For this review, use the dimensioned drawing (mm, ordinates from the lowest corner) and the shaded views. Give positions to 0.01 mm unless a question says otherwise; leave off trailing zeros. Loops run counter-clockwise (first coordinate to the right, second up) from the corner with the lowest first, then second, coordinate; pieces in that order, holes last. Notation, with made-up numbers: (35, -22.75) -> (58, -22.75) arc R16 cw to (58, -7.75) -> close; hole circle Ø11 at (41, -37). An arc over 180 degrees is marked (long way). Use a Markdown table: item, result. Add a question column.
1. For pin 1 Ø2 at (y, z) = (3, 0.5) entering from -X; pin 2 Ø1.5 at (x, z) = (3, 3) entering from -Y; pin 3 Ø2 at (y, z) = (4, 2.5) entering from -X, all flat-tipped, find the tip position at first contact; note any pin that passes through.
2. Add section C-C (z = 2.25). State the section outline as (x, y) points, and give its area (3 significant figures).
3. Add section A-A (y = 6.75). State the section outline as (x, z) points, and give its area (3 significant figures).
4. Draft analysis for pull direction Y (two halves, no side actions). For the marked faces 1, 2 and 3, state which applies: pulls with the +Y half, pulls with the -Y half, needs draft (parallel to the pull), parting line crosses it, or undercut.
5. To check wall thickness, follow line 1 (Y direction, x = 6.75, z = 1.55); line 2 (Y direction, x = 9.5, z = 3.25); line 3 (X direction, y = 5.75, z = 3.05). State the ranges of each line that lie inside material, in increasing order.
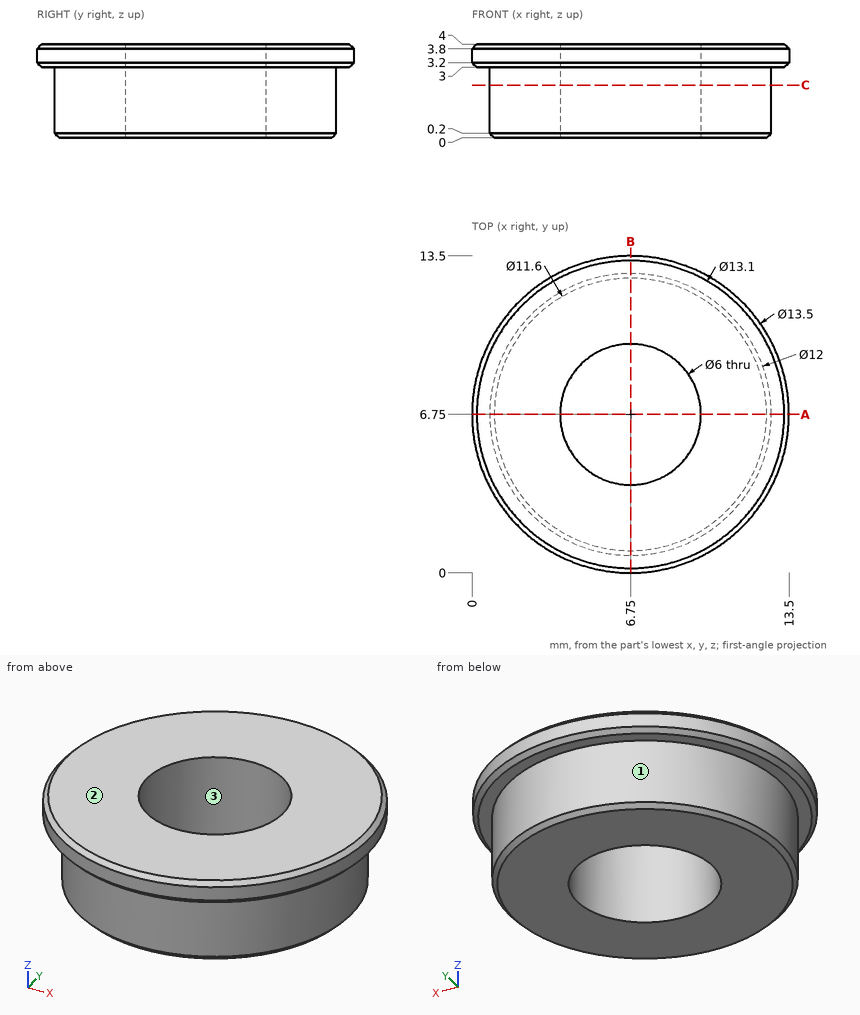
Taken from the geometry:
| question | item | result |
|---|---|---|
| 1 | pin 1 | stops at x = 1.42 |
| 1 | pin 2 | stops at y = 0.72 |
| 1 | pin 3 | stops at x = 0.31 |
| 2 | outline | circle Ø12 at (6.75, 6.75); hole circle Ø6 at (6.75, 6.75) |
| 2 | area | 84.8 mm^2 |
| 3 | outline | (0, 3.2) -> (0.2, 3) -> (0.75, 3) -> (0.75, 0.2) -> (0.95, 0) -> (3.75, 0) -> (3.75, 4) -> (0.2, 4) -> (0, 3.8) -> close; (9.75, 0) -> (12.55, 0) -> (12.75, 0.2) -> (12.75, 3) -> (13.3, 3) -> (13.5, 3.2) -> (13.5, 3.8) -> (13.3, 4) -> (9.75, 4) -> close |
| 3 | area | 25.4 mm^2 |
| 4 | face 1 | parting line crosses it |
| 4 | face 2 | needs draft |
| 4 | face 3 | undercut |
| 5 | line 1 | y = 0.75 to 3.75, 9.75 to 12.75 |
| 5 | line 2 | y = 0.59 to 5.55, 7.95 to 12.91 |
| 5 | line 3 | x = 0.23 to 3.92, 9.58 to 13.27 |
